Answer from the drawing. Dimensions are ordinates in mm from the lowest x, y and z of the part. Coordinates: 2 decimals unless noted, no trailing zeros. Write each loop counter-clockwise with the first axis right and the second up, starting at its lowest first coordinate (ties: lowest second). Pieces come first, ordered by that corner, then holes. Notation, with made-up numbers: (68, 6.5) - (90, 6.5) arc R17 ccw to (90, 28.5) - close; hole circle Ø1 at (-32, 87). An arc over 180 degrees is marked (long way). Return JSON: item names as keys, results as strings.
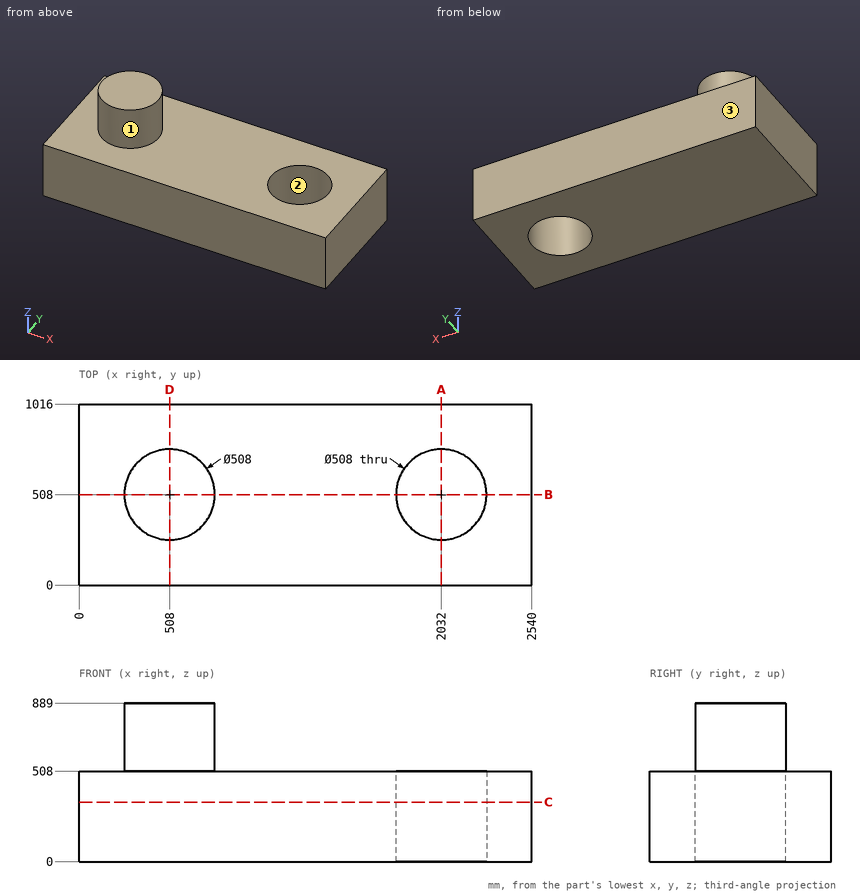
(1) A cutting plane is placed at C-C (z = 333.5). Determine the outline of the cut face in (x, y), and give its area (3 significant figures).
Answer:
{"outline": "(0, 0) - (2540, 0) - (2540, 1016) - (0, 1016) - close; hole circle Ø508 at (2032, 508)", "area": "2,380,000 mm²"}
(2) A cutting plane is placed at A-A (x = 2032). Determine the outline of the cut face in (y, z).
Answer:
{"outline": "(0, 0) - (254, 0) - (254, 508) - (0, 508) - close; (762, 0) - (1016, 0) - (1016, 508) - (762, 508) - close"}
(3) Determine the mould class of the marked faces 1, 2 and 3 for opening direction X: +X half, -X half, draft (parallel to the pull), parting line (faces both ways), or undercut.
Answer:
{"face 1": "parting line", "face 2": "undercut", "face 3": "draft"}
(4) Straight lines are drawn through the part: line 1 (Y direction, x = 2032, z = 343); line 2 (Z direction, x = 598.5, y = 882); line 3 (X direction, y = 668.5, z = 505). For each, find the intervals that lie inside material, in ascending order. Write a range as from..to.
Answer:
{"line 1": "0..254, 762..1016", "line 2": "0..508", "line 3": "0..1835.14, 2228.86..2540"}
(5) A cutting plane is placed at D-D (x = 508). Determine the outline of the cut face in (y, z), and give its area (3 significant figures).
Answer:
{"outline": "(0, 0) - (1016, 0) - (1016, 508) - (762, 508) - (762, 889) - (254, 889) - (254, 508) - (0, 508) - close", "area": "710,000 mm²"}
(6) Flat-ended cylindrical pins translate along their axes: P1, Ø2, axis at x = 376, z = 640.5, coming from the -Y side; P2, Ø4, axis at x = 343.5, z = 643, coming from the -Y side. Find the tip coordinate at first contact, or state that the pin passes through.
Answer:
{"P1": "y = 290.39", "P2": "y = 312.78"}
(7) A cutting plane is placed at B-B (y = 508). Determine the outline of the cut face in (x, z).
Answer:
{"outline": "(0, 0) - (1778, 0) - (1778, 508) - (762, 508) - (762, 889) - (254, 889) - (254, 508) - (0, 508) - close; (2286, 0) - (2540, 0) - (2540, 508) - (2286, 508) - close"}
